```python
from build123d import *

# Parameters (mm, degrees)
SKETCH1_W                                            = 65
SKETCH1_H                                            = 55
BOSS_EXTRUDE1_DEPTH                                  = 16
CBORE_SLOT_FOR_M6_HEX_SOCKET_HEAD_CAP_SC_D           = 6.6
CBORE_SLOT_FOR_M6_HEX_SOCKET_HEAD_CAP_SC_CBORE_D     = 11
CBORE_SLOT_FOR_M6_HEX_SOCKET_HEAD_CAP_SC_CBORE_DEPTH = 7
F_6_0MM_DOWEL_HOLE1_D                                = 6
SKETCH23_R                                           = 13
CUT_EXTRUDE2_DEPTH                                   = 8
SKETCH24_R                                           = 10
CUT_EXTRUDE3_DEPTH                                   = 86.521927013


with BuildPart() as part:
    # Sketch1 → Boss-Extrude1 (new body)
    with BuildSketch(Plane(origin=(0, 0, 0), x_dir=(1, 0, 0), z_dir=(0, 1, 0))):
        with Locations((32.5, 27.5)):
            Rectangle(SKETCH1_W, SKETCH1_H)
    extrude(amount=BOSS_EXTRUDE1_DEPTH)

    # CBORE SLOT for M6 Hex Socket Head Cap Screw1 (through all)
    with Locations(Plane(origin=(0, 16, 0), x_dir=(1, 0, 0), z_dir=(0, 1, 0))):
        with Locations((10, 45), (55, 45), (55, 10), (10, 10)):
            CounterBoreHole(CBORE_SLOT_FOR_M6_HEX_SOCKET_HEAD_CAP_SC_D / 2, CBORE_SLOT_FOR_M6_HEX_SOCKET_HEAD_CAP_SC_CBORE_D / 2, CBORE_SLOT_FOR_M6_HEX_SOCKET_HEAD_CAP_SC_CBORE_DEPTH)

    # Ø6.0mm Dowel Hole1 (through all)
    with Locations(Plane(origin=(0, 16, 0), x_dir=(1, 0, 0), z_dir=(0, 1, 0))):
        with Locations((10.078116325, 27.5), (55, 27.5)):
            Hole(F_6_0MM_DOWEL_HOLE1_D / 2)

    # Sketch23 → Cut-Extrude2 (cut)
    with BuildSketch(Plane.XZ):
        with BuildLine():
            ThreePointArc((45.5, -27.5), (32.5, -40.5), (19.5, -27.5))
            Line((19.5, -27.5), (19.5, -55))
            Line((19.5, -55), (45.5, -55))
            Line((45.5, -55), (45.5, -27.5))
        make_face()
        with Locations((32.5, -27.5)):
            Circle(SKETCH23_R)
    extrude(amount=-CUT_EXTRUDE2_DEPTH, mode=Mode.SUBTRACT)

    # Sketch24 → Cut-Extrude3 (cut, through all)
    with BuildSketch(Plane.XZ.offset(-8)):
        with Locations((32.5, -27.5)):
            Circle(SKETCH24_R)
        with BuildLine():
            Line((42.5, -55), (42.5, -27.5))
            ThreePointArc((42.5, -27.5), (32.5, -37.5), (22.5, -27.5))
            Line((22.5, -27.5), (22.5, -55))
            Line((22.5, -55), (42.5, -55))
        make_face()
    extrude(amount=-CUT_EXTRUDE3_DEPTH, mode=Mode.SUBTRACT)


solid = part.part
```
Part model, mm, in its own coordinate system. A direction names the side the tool comes from. Round coordinates to 2 decimals unless told otherwise and drop trailing zeros. Loops run counter-clockwise (first coordinate to the right, second up) from the corner with the lowest first, then second, coordinate; pieces in that order, holes last. Notation, with made-up numbers: (36.25, 60.25) -> (57.25, 60.25) arc R19 ccw to (57.25, 89.25) -> close; hole circle Ø8 at (83, 46). An arc over 180 degrees is marked (long way). Use CSV: the item, a comma, the result in double quotes. Start each with the question number.
1) Wall check: L1, parallel to Z at x = 55, y = 2; L2, parallel to X at y = 5, z = -27.5; L3, parallel to X at y = 10.5, z = -14. Give the ranges that are in metal, low to high. Write a range as [from, to].
2) Cut at C-C, the plane y = 2.75. Write the cut outline in (x, z).
3) Cut at B-B, the plane x = 55. Write the cut outline in (y, z).
4) Pull direction Z, two halves, no side cores. Call faces 4 (the cylindrical face through (32.7, 11.9, -17.5)), 5 (the flat face through (45.5, 4, -41)), 6 (the cylindrical face through (9.284, 12.549, -50.453)): +Z half, -Z half, draft (parallel to the pull), parting line (faces both ways), or undercut.
5) Cut at A-A, the plane z = -10. Write the cut outline in (x, y), plus the area to 3 significant figures.
6) Which spindle directions (+Z, -Z, +X, -X, +Y, -Y) get a long thin tool onto all of the face, cutting with end or side? Do faces 1 (the flat face through (22, 8, -32)), 2 (the cylindrical face through (10.43, 4.44, -48.27)), 3 (the cylindrical face through (49.505, 12.549, -10.242)). Say none if no direction does.
7) Cut at D-D, the plane z = -45. Write the cut outline in (x, y), plus the area to 3 significant figures.
8) Drop a flat-ended pin along its axis: P1, Ø10, axis at x = 55, z = -10, coming from the +Y side. Give the stop position or say it passes through.
Determined:
1,L1,"z = [-55, -48.3], [-41.7, -30.5], [-24.5, -13.3], [-6.7, 0]"
1,L2,"x = [0, 7.08], [13.08, 19.5], [45.5, 52], [58, 65]"
1,L3,"x = [0, 6.23], [13.77, 51.23], [58.77, 65]"
2,outline,"(0, -55) -> (19.5, -55) -> (19.5, -27.5) arc R13 cw to (45.5, -27.5) -> (45.5, -55) -> (65, -55) -> (65, 0) -> (0, 0) -> close; hole circle Ø6.6 at (10, -45); hole circle Ø6.6 at (10, -10); hole circle Ø6 at (10.08, -27.5); hole circle Ø6.6 at (55, -45); hole circle Ø6.6 at (55, -10); hole circle Ø6 at (55, -27.5)"
3,outline,"(0, -55) -> (16, -55) -> (16, -50.5) -> (9, -50.5) -> (9, -48.3) -> (0, -48.3) -> close; (0, -41.7) -> (9, -41.7) -> (9, -39.5) -> (16, -39.5) -> (16, -30.5) -> (0, -30.5) -> close; (0, -24.5) -> (16, -24.5) -> (16, -15.5) -> (9, -15.5) -> (9, -13.3) -> (0, -13.3) -> close; (0, -6.7) -> (9, -6.7) -> (9, -4.5) -> (16, -4.5) -> (16, 0) -> (0, 0) -> close"
4,face 4,"-Z half"
4,face 5,"draft"
4,face 6,"undercut"
5,outline,"(0, 0) -> (6.7, 0) -> (6.7, 9) -> (4.5, 9) -> (4.5, 16) -> (0, 16) -> close; (13.3, 0) -> (51.7, 0) -> (51.7, 9) -> (49.5, 9) -> (49.5, 16) -> (15.5, 16) -> (15.5, 9) -> (13.3, 9) -> close; (58.3, 0) -> (65, 0) -> (65, 16) -> (60.5, 16) -> (60.5, 9) -> (58.3, 9) -> close"
5,area,"767 mm2"
6,face 1,"-Z, -Y"
6,face 2,"+Y, -Y"
6,face 3,"+Y"
7,outline,"(0, 0) -> (6.7, 0) -> (6.7, 9) -> (4.5, 9) -> (4.5, 16) -> (0, 16) -> close; (13.3, 0) -> (19.5, 0) -> (19.5, 8) -> (22.5, 8) -> (22.5, 16) -> (15.5, 16) -> (15.5, 9) -> (13.3, 9) -> close; (42.5, 8) -> (45.5, 8) -> (45.5, 0) -> (51.7, 0) -> (51.7, 9) -> (49.5, 9) -> (49.5, 16) -> (42.5, 16) -> close; (58.3, 0) -> (65, 0) -> (65, 16) -> (60.5, 16) -> (60.5, 9) -> (58.3, 9) -> close"
7,area,"399 mm2"
8,P1,"stops at y = 9"
